Could you check a few things on this model? Use its own coordinates, in mm. A direction names the side the tool comes from. Give positions to 0.01 mm unless a question says otherwise; leave off trailing zeros. Loops run counter-clockwise (first coordinate to the right, second up) from the corner with the lowest first, then second, coordinate; pieces in that order, holes last. Notation, with made-up numbers: (57.5, 5.5) -> (63.5, 5.5) arc R29 ccw to (63.5, 36.5) -> close; hole circle Ø9 at (-20, 21.25). An arc over 180 degrees is marked (long way). Put each result on its own line as item: value.
```python
from build123d import *

# Parameters (mm, degrees)
SKETCH2_R           = 60.625
SKETCH2_R_2         = 45
BOSS_EXTRUDE1_DEPTH = 4
SKETCH4_R           = 49
SKETCH4_R_2         = 45
BOSS_EXTRUDE2_DEPTH = 52
SKETCH5_W           = 8
SKETCH5_H           = 38
SKETCH5_W_2         = 15
SKETCH5_H_2         = 8
BOSS_EXTRUDE3_DEPTH = 13
SKETCH6_W           = 10
SKETCH6_H           = 24
CUT_EXTRUDE2_DEPTH  = 8
SKETCH7_R           = 5
CUT_EXTRUDE3_DEPTH  = 110.441337026
SKETCH8_R           = 1.3
CUT_EXTRUDE4_DEPTH  = 7.2
BOSS_EXTRUDE4_DEPTH = 4
SKETCH10_R          = 1.5
CUT_EXTRUDE5_DEPTH  = 103.404986506
FILLET1_R           = 1


with BuildPart() as part:
    # Sketch2 → Boss-Extrude1 (new body)
    with BuildSketch(Plane(origin=(0, 0, 0), x_dir=(1, 0, 0), z_dir=(0, 1, 0))):
        with Locations(Location((0, 0, 0), (0, 0, 270))):
            Circle(SKETCH2_R)
        with Locations(Location((0, 0, 0), (0, 0, 270))):
            Circle(SKETCH2_R_2, mode=Mode.SUBTRACT)
    extrude(amount=BOSS_EXTRUDE1_DEPTH)

    # Sketch4 → Boss-Extrude2 (add)
    with BuildSketch(Plane(origin=(0, 4, 0), x_dir=(1, 0, 0), z_dir=(0, 1, 0))):
        with Locations(Location((0, 0.954313472, 0), (0, 0, 90))):
            Circle(SKETCH4_R)
        with Locations(Location((0, 0, 0), (0, 0, 270))):
            Circle(SKETCH4_R_2, mode=Mode.SUBTRACT)
    extrude(amount=BOSS_EXTRUDE2_DEPTH)

    # Sketch5 → Boss-Extrude3 (add, symmetric)
    with BuildSketch(Plane.XY):
        with Locations((15.25, 19)):
            Rectangle(SKETCH5_W, SKETCH5_H)
        with Locations((-39.25, 34)):
            Rectangle(SKETCH5_W_2, SKETCH5_H_2)
    extrude(amount=BOSS_EXTRUDE3_DEPTH, both=True)


with BuildPart() as boss_extrude3_piece_1:
    # of the separate pieces the step leaves, piece 1, a body of its own (boss_extrude3_pieces)
    add(part.part.solids().sort_by_distance((0, 0, 60.625))[0])

    # Sketch7 → Cut-Extrude3 (cut, through all)
    with BuildSketch(Plane.ZY.offset(-11.25)):
        with Locations((0, 14)):
            Circle(SKETCH7_R)
    extrude(amount=-CUT_EXTRUDE3_DEPTH, mode=Mode.SUBTRACT)


with BuildPart() as boss_extrude3_piece_2:
    # of the separate pieces the step leaves, piece 2, a body of its own (boss_extrude3_pieces)
    add(part.part.solids().sort_by_distance((11.25, 0, -13))[0])

    # Sketch6 → Cut-Extrude2 (cut)
    with BuildSketch(Plane.ZY.offset(-11.25)):
        with Locations((0, 17)):
            Rectangle(SKETCH6_W, SKETCH6_H)
    extrude(amount=-CUT_EXTRUDE2_DEPTH, mode=Mode.SUBTRACT)


with BuildPart() as cut_extrude4_tool:
    # Sketch8 → Cut-Extrude4 (new body)
    with BuildSketch(Plane(origin=(0, 38, 0), x_dir=(1, 0, 0), z_dir=(0, 1, 0))):
        with Locations(Location((-34.25, 5, 0), (0, 0, 270))):
            Circle(SKETCH8_R)
        with Locations(Location((-34.25, -5, 0), (0, 0, 270))):
            Circle(SKETCH8_R)
        with Locations(Location((13.75, -5, 0), (0, 0, 270))):
            Circle(SKETCH8_R)
        with Locations(Location((13.75, 5, 0), (0, 0, 270))):
            Circle(SKETCH8_R)
    extrude(amount=-CUT_EXTRUDE4_DEPTH)


with BuildPart() as boss_extrude3_piece_1_1:
    add(boss_extrude3_piece_1.part)

    # Cut-Extrude4: cut by cut_extrude4_tool
    add(cut_extrude4_tool.part, mode=Mode.SUBTRACT)



with BuildPart() as boss_extrude3_piece_2_1:
    add(boss_extrude3_piece_2.part)

    # Cut-Extrude4: cut by cut_extrude4_tool
    add(cut_extrude4_tool.part, mode=Mode.SUBTRACT)


with BuildPart() as boss_extrude3_piece_1_2:
    add(boss_extrude3_piece_1_1.part)

    add(boss_extrude3_piece_2_1.part)  # Boss-Extrude4 merges Boss-Extrude3 piece 2
    # Sketch9 → Boss-Extrude4 (add)
    with BuildSketch(Plane.XZ):
        with BuildLine():
            Line((11.25, 13), (25.249838503, 37.248431585))
            ThreePointArc((25.249838503, 37.248431585), (45, 0), (25.249838503, -37.248431585))
            Line((25.249838503, -37.248431585), (11.25, -13))
            Line((11.25, -13), (11.25, 13))
        make_face()
        with BuildLine():
            Line((24.25, 19.516660498), (27.361802413, 24.906460381))
            ThreePointArc((27.361802413, 24.906460381), (37, 0), (27.361802413, -24.906460381))
            Line((27.361802413, -24.906460381), (24.25, -19.516660498))
            Line((24.25, -19.516660498), (24.25, 19.516660498))
        make_face(mode=Mode.SUBTRACT)
    extrude(amount=-BOSS_EXTRUDE4_DEPTH)

    # Sketch10 → Cut-Extrude5 (cut, through all)
    with BuildSketch(Plane.XZ):
        with Locations(Location((54.5, 0, 0), (0, 0, 270))):
            Circle(SKETCH10_R)
        with Locations(Location((0, -54.5, 0), (0, 0, 270))):
            Circle(SKETCH10_R)
        with Locations(Location((-54.5, 0, 0), (0, 0, 270))):
            Circle(SKETCH10_R)
        with Locations(Location((0, 54.5, 0), (0, 0, 270))):
            Circle(SKETCH10_R)
    extrude(amount=-CUT_EXTRUDE5_DEPTH, mode=Mode.SUBTRACT)

    # Fillet1
    fillet1_edges = [boss_extrude3_piece_1_2.edges().sort_by_distance(p)[0] for p in [
        (0, 4, -60.625),
        (0, 4, 48.045686528),
    ]]
    fillet(fillet1_edges, radius=FILLET1_R)


solid = boss_extrude3_piece_1_2.part
```
1. Thinking about a two-plate mould opening in Y: for faces 1 (the face through (15, 5, 0)), 2 (the face through (25.8, 2, -22.2)), 3 (the face through (-13, 4, 48)), which applies, pulls with the +Y half, pulls with the -Y half, needs draft (parallel to the pull), parting line crosses it, or undercut?
Recorded:
face 1: undercut
face 2: needs draft
face 3: pulls with the +Y half
2. If we section it at A-A (y = 27): List the corners of the cut face in (x, z) for me, then the cut area to 3 significant figures.
Recorded:
outline: circle Ø98 at (0, -0.95); (11.25, -13) -> (19.25, -13) -> (19.25, -5) -> (11.25, -5) -> close; (11.25, 5) -> (19.25, 5) -> (19.25, 13) -> (11.25, 13) -> close; hole circle Ø90 at (0, 0)
area: 1,310 mm^2
3. I need wall thicknesses on line 1 (X direction, y = 2.7, z = 0) (3 decimals); line 2 (Z direction, x = -1, y = 31); line 3 (X direction, y = 3.5, z = -17.5). Which ranges of each line are inside material? Lowest first, please.
Recorded:
line 1: x = -60.625 to -56, -53 to -45, 11.25 to 24.25, 37 to 53, 56 to 60.625
line 2: z = -49.94 to -44.99, 44.99 to 48.04
line 3: x = -57.9 to -41.46, 13.85 to 24.25, 32.6 to 57.9
4. If we section it at C-C (z = -15): Count the separate pieces of the cut face and the enclosed holes in it, then the cut area to 3 significant figures.
Recorded:
separate pieces: 3
enclosed holes: 0
area: 682 mm^2
5. For faces 4 (the face through (15, 17, -5)), 5 (the face through (18.348, 1.972, -25.294)), 6 (the face through (47, 17, -4)), 7 (the face through (19.25, 21, -6)), which set-ups out of +Z, -Z, +X, -X, +Y, -Y let a thin tool reach every point of the face, with its end or its side?
Recorded:
face 4: none
face 5: +Y, -Y
face 6: +X
face 7: +Y
6. I'm going to push flat-ended pins straight in: pin 1 (6.5 mm diameter, centred on x = 15.5, y = 26, fed in from -Z); pin 2 (8 mm diameter, centred on x = 6, z = 16.5, fed in from -Y); pin 3 (3 mm diameter, centred on y = 45.5, z = -23, fed in from -X); pin 4 (3.5 mm diameter, centred on x = 0, z = -54.5, fed in from -Y). Where does each tip first touch, or does it pass through?
Recorded:
pin 1: stops at z = -48.4
pin 2: passes through
pin 3: stops at x = -44.48
pin 4: stops at y = 0
7. If we section it at B-B (y = 14): List the corners of the cut face in (x, z) for me, then the cut area to 3 significant figures.
Recorded:
outline: (11.25, -13) -> (19.25, -13) -> (19.25, -5) -> (11.25, -5) -> close; (11.25, 5) -> (19.25, 5) -> (19.25, 13) -> (11.25, 13) -> close; (44.72, -5) arc R45 cw (long way) to (44.72, 5) -> (48.64, 5) arc R49 ccw (long way) to (48.83, -5) -> close
area: 1,270 mm^2
